Drawing for the job (mm, zero at the part's lowest x, y, z). A direction names the side the tool comes from. Coordinates: 2 decimals unless noted, no trailing zeros. Write each loop counter-clockwise with the first axis right and the second up, starting at its lowest first coordinate (ties: lowest second). Pieces come first, ordered by that corner, then holes. Notation, with made-up numbers: (51.5, 73.5) -> (96.5, 73.5) arc R25 ccw to (96.5, 106.5) -> close; hole circle Ø5 at (65, 29.5). An arc over 180 degrees is marked (long way). Write each question's results on one line, items separated by ' | '. Start each with the question number.
Q1. Tool access for the marked faces 1, 2, 3, 4 and 5: list every direction of +Z, -Z, +X, -X, +Y, -Y with a clear straight run to the whole face (end or side of a thin tool).
Q2. Saw through at D-D on y = 87. Give the cut face in (x, z), and give its area (3 significant figures).
Q3. Drop flat-ended pins along their axis: pin 1 Ø4 at (x, z) = (81, 5.5) entering from -Y; pin 2 Ø4 at (y, z) = (70.5, 3) entering from +X; pin 3 Ø4 at (y, z) = (26, 4.5) entering from -X. Give the stop position or say it passes through.
Q4. Saw through at A-A on x = 82. Give the cut face in (y, z), and give its area (3 significant figures).
Q5. Saw through at C-C on z = 4.5. Give the cut face in (x, y), and give its area (3 significant figures).
Q6. Drill centre lines: line 1 (Y direction, x = 6, z = 3.5); line 2 (X direction, y = 63.5, z = 6); line 3 (Y direction, x = 4, z = 4). Where is each one in solid material? Low to high.
Q7. Saw through at B-B on y = 51.5. Give the cut face in (x, z).
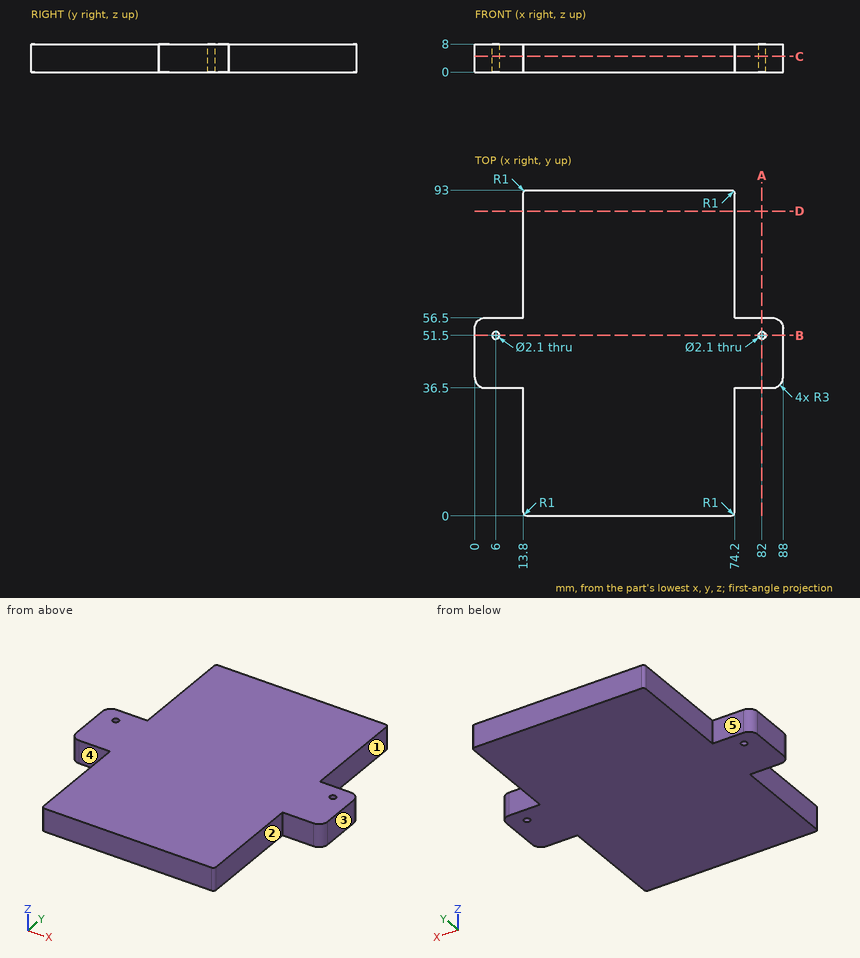
Returned:
1) face 1: +Z, -Z, +X, +Y | face 2: +Z, -Z, +X, -Y | face 3: +Z, -Z, +X, +Y, -Y | face 4: +Z, -Z, -X, -Y | face 5: +Z, -Z, -X, +Y
2) outline: (13.8, 0) -> (74.2, 0) -> (74.2, 8) -> (13.8, 8) -> close | area: 483 mm2
3) pin 1: stops at y = 36.5 | pin 2: stops at x = 74.2 | pin 3: stops at x = 13.8
4) outline: (36.5, 0) -> (50.45, 0) -> (50.45, 8) -> (36.5, 8) -> close; (52.55, 0) -> (56.5, 0) -> (56.5, 8) -> (52.55, 8) -> close | area: 143 mm2
5) outline: (0, 39.5) arc R3 ccw to (3, 36.5) -> (13.8, 36.5) -> (13.8, 1) arc R1 ccw to (14.8, 0) -> (73.2, 0) arc R1 ccw to (74.2, 1) -> (74.2, 36.5) -> (85, 36.5) arc R3 ccw to (88, 39.5) -> (88, 53.5) arc R3 ccw to (85, 56.5) -> (74.2, 56.5) -> (74.2, 92) arc R1 ccw to (73.2, 93) -> (14.8, 93) arc R1 ccw to (13.8, 92) -> (13.8, 56.5) -> (3, 56.5) arc R3 ccw to (0, 53.5) -> close; hole circle Ø2.1 at (6, 51.5); hole circle Ø2.1 at (82, 51.5) | area: 6,150 mm2
6) line 1: y = 36.5 to 50.45, 52.55 to 56.5 | line 2: x = 13.8 to 74.2 | line 3: y = 36.5 to 56.5
7) outline: (0, 0) -> (4.95, 0) -> (4.95, 8) -> (0, 8) -> close; (7.05, 0) -> (80.95, 0) -> (80.95, 8) -> (7.05, 8) -> close; (83.05, 0) -> (88, 0) -> (88, 8) -> (83.05, 8) -> close
